Check sheet for the modelled part. Datum: model origin and axes. Units: mm. A direction names the side the tool comes from. Round coordinates to 2 decimals unless told otherwise and drop trailing zeros. Loops run counter-clockwise (first coordinate to the right, second up) from the corner with the lowest first, then second, coordinate; pieces in that order, holes last. Notation, with made-up numbers: (3, 57) -> (53, 57) arc R31 cw to (53, 88) -> close; hole circle Ø4 at (39.5, 83). An arc over 180 degrees is marked (long way). One line per question, with ' | ' between items.
```python
from build123d import *

# Parameters (mm, degrees)
SKETCH1_W           = 31.5
SKETCH1_H           = 27
SKETCH1_R           = 1.5625
SKETCH1_W_2         = 12
SKETCH1_H_2         = 8
BOSS_EXTRUDE1_DEPTH = 2
SKETCH1_3_W         = 12
SKETCH1_3_H         = 8
BOSS_EXTRUDE2_DEPTH = 1
SKETCH2_R           = 1.003384187
BOSS_EXTRUDE3_DEPTH = 0.1


with BuildPart() as part:
    # Sketch1 → Boss-Extrude1 (new body)
    with BuildSketch(Plane.XY):
        Rectangle(SKETCH1_W, SKETCH1_H)
        with Locations((12.75, -10.5)):
            Circle(SKETCH1_R, mode=Mode.SUBTRACT)
        with Locations((12.75, 10.5)):
            Circle(SKETCH1_R, mode=Mode.SUBTRACT)
        with Locations((-12.75, -10.5)):
            Circle(SKETCH1_R, mode=Mode.SUBTRACT)
        with Locations((-12.75, 10.5)):
            Circle(SKETCH1_R, mode=Mode.SUBTRACT)
        Rectangle(SKETCH1_W_2, SKETCH1_H_2, mode=Mode.SUBTRACT)
        Rectangle(SKETCH1_W_2, SKETCH1_H_2)
    extrude(amount=BOSS_EXTRUDE1_DEPTH)

    # Sketch1_3 → Boss-Extrude2 (add)
    with BuildSketch(Plane.XY):
        Rectangle(SKETCH1_3_W, SKETCH1_3_H)
    extrude(amount=-BOSS_EXTRUDE2_DEPTH)

    # Sketch2 → Boss-Extrude3 (add)
    with BuildSketch(Plane(origin=(0, 0, -1), x_dir=(-1, 0, 0), z_dir=(0, 0, -1))):
        with Locations(Location((0, 0, 0), (0, 0, 180))):
            Circle(SKETCH2_R)
    extrude(amount=BOSS_EXTRUDE3_DEPTH)


solid = part.part
```
(1) Scan lines: probe 1 along Y at (x, z) = (12.75, 1.35); probe 2 along X at (y, z) = (-10, 1); probe 3 along X at (y, z) = (-11.5, 1.85). Record each from-to range of solid material in increasing order.
Answer:
probe 1: y = -13.5 to -12.06, -8.94 to 8.94, 12.06 to 13.5 | probe 2: x = -15.75 to -14.23, -11.27 to 11.27, 14.23 to 15.75 | probe 3: x = -15.75 to -13.95, -11.55 to 11.55, 13.95 to 15.75
(2) Set-up check for faces 1 (the face through (-6, -0.1, -0.5)), 2 (the face through (-0.1, -4, -0.5)), 3 (the face through (6, -0.1, -0.5)): record each of +Z, -Z, +X, -X, +Y, -Y from which the full face is reachable in a straight line by a thin tool's end or side.
Answer:
face 1: -Z, -X, +Y, -Y | face 2: -Z, +X, -X, -Y | face 3: -Z, +X, +Y, -Y
(3) Go/stop test with flat-tipped pins: pin 1 (2.5 mm diameter, centred on x = 12.75, y = 10.5, fed in from +Z) (3 decimals); pin 2 (3.5 mm diameter, centred on x = 12.75, y = -10.5, fed in from -Z); pin 3 (0.8 mm diameter, centred on x = 3, z = -0.5, fed in from +Y); pin 4 (0.5 mm diameter, centred on x = 1, z = -0.5, fed in from -Y). Record where each tip stops, or that it passes through.
Answer:
pin 1: passes through | pin 2: stops at z = 0 | pin 3: stops at y = 4 | pin 4: stops at y = -4
(4) Mould release check, pull along X, two halves, no side actions. Record for faces 4 (the face through (-11.26, -10.03, 0.99)), 5 (the face through (0, 6, 0)), 6 (the face through (15.75, 0, 1)), 7 (the face through (14.24, -10.03, 0.99)): +X half, -X half, draft (parallel to the pull), parting line (faces both ways), or undercut.
Answer:
face 4: undercut | face 5: draft | face 6: +X half | face 7: undercut
(5) Sectioned sample at D-D, the plane x = 0. Record the cut outline in (y, z).
Answer:
outline: (-13.5, 0) -> (-4, 0) -> (-4, -1) -> (-1, -1) -> (-1, -1.1) -> (1, -1.1) -> (1, -1) -> (4, -1) -> (4, 0) -> (13.5, 0) -> (13.5, 2) -> (-13.5, 2) -> close
(6) Sectioned sample at B-B, the plane x = -12.75. Record the cut outline in (y, z), and give its area (3 significant figures).
Answer:
outline: (-13.5, 0) -> (-12.06, 0) -> (-12.06, 2) -> (-13.5, 2) -> close; (-8.94, 0) -> (8.94, 0) -> (8.94, 2) -> (-8.94, 2) -> close; (12.06, 0) -> (13.5, 0) -> (13.5, 2) -> (12.06, 2) -> close | area: 41.5 mm2
(7) Sectioned sample at C-C, the plane z = 0.8. Count the separate pieces of the cut face and the enclosed holes in it, and give its area (3 significant figures).
Answer:
separate pieces: 1 | enclosed holes: 4 | area: 820 mm2
(8) Sectioned sample at A-A, the plane y = 10.5. Record the cut outline in (x, z).
Answer:
outline: (-15.75, 0) -> (-14.31, 0) -> (-14.31, 2) -> (-15.75, 2) -> close; (-11.19, 0) -> (11.19, 0) -> (11.19, 2) -> (-11.19, 2) -> close; (14.31, 0) -> (15.75, 0) -> (15.75, 2) -> (14.31, 2) -> close
